```python
from build123d import *

# Parameters (mm, degrees)
ESBO_O1_W                = 9
ESBO_O1_H                = 9
ESBO_O1_R                = 8
RESSALTO_EXTRUS_O4_DEPTH = 500


with BuildPart() as part:
    # Esboço1 → Ressalto-extrusão4 (new body)
    with BuildSketch(Plane.XY):
        with BuildLine():
            Line((-4.5, 22.5), (-22.5, 22.5))
            Line((-22.5, 22.5), (-22.5, 4.5))
            Line((-22.5, 4.5), (-17.5, 4.5))
            Line((-17.5, 4.5), (-17.5, 5))
            Line((-17.5, 5), (-22, 5))
            Line((-22, 5), (-22, 12.5))
            Line((-22, 12.5), (-13.207106781, 12.5))
            Line((-13.207106781, 12.5), (-6.707685904, 6.000579123))
            ThreePointArc((-6.707685904, 6.000579123), (-9, 0), (-6.707685904, -6.000579123))
            Line((-6.707685904, -6.000579123), (-13.207106781, -12.5))
            Line((-13.207106781, -12.5), (-22, -12.5))
            Line((-22, -12.5), (-22, -5))
            Line((-22, -5), (-17.5, -5))
            Line((-17.5, -5), (-17.5, -4.5))
            Line((-17.5, -4.5), (-22.5, -4.5))
            Line((-22.5, -4.5), (-22.5, -22.5))
            Line((-22.5, -22.5), (-4.5, -22.5))
            Line((-4.5, -22.5), (-4.5, -17.5))
            Line((-4.5, -17.5), (-5, -17.5))
            Line((-5, -17.5), (-5, -22))
            Line((-5, -22), (-12.5, -22))
            Line((-12.5, -22), (-12.5, -13.207106781))
            Line((-12.5, -13.207106781), (-6.000579123, -6.707685904))
            ThreePointArc((-6.000579123, -6.707685904), (0, -9), (6.000579123, -6.707685904))
            Line((6.000579123, -6.707685904), (12.5, -13.207106781))
            Line((12.5, -13.207106781), (12.5, -22))
            Line((12.5, -22), (5, -22))
            Line((5, -22), (5, -17.5))
            Line((5, -17.5), (4.5, -17.5))
            Line((4.5, -17.5), (4.5, -22.5))
            Line((4.5, -22.5), (22.5, -22.5))
            Line((22.5, -22.5), (22.5, -4.5))
            Line((22.5, -4.5), (17.5, -4.5))
            Line((17.5, -4.5), (17.5, -5))
            Line((17.5, -5), (22, -5))
            Line((22, -5), (22, -12.5))
            Line((22, -12.5), (13.207106781, -12.5))
            Line((13.207106781, -12.5), (6.707685904, -6.000579123))
            ThreePointArc((6.707685904, -6.000579123), (9, 0), (6.707685904, 6.000579123))
            Line((6.707685904, 6.000579123), (13.207106781, 12.5))
            Line((13.207106781, 12.5), (22, 12.5))
            Line((22, 12.5), (22, 5))
            Line((22, 5), (17.5, 5))
            Line((17.5, 5), (17.5, 4.5))
            Line((17.5, 4.5), (22.5, 4.5))
            Line((22.5, 4.5), (22.5, 22.5))
            Line((22.5, 22.5), (4.5, 22.5))
            Line((4.5, 22.5), (4.5, 17.5))
            Line((4.5, 17.5), (5, 17.5))
            Line((5, 17.5), (5, 22))
            Line((5, 22), (12.5, 22))
            Line((12.5, 22), (12.5, 13.207106781))
            Line((12.5, 13.207106781), (6.000579123, 6.707685904))
            ThreePointArc((6.000579123, 6.707685904), (0, 9), (-6.000579123, 6.707685904))
            Line((-6.000579123, 6.707685904), (-12.5, 13.207106781))
            Line((-12.5, 13.207106781), (-12.5, 22))
            Line((-12.5, 22), (-5, 22))
            Line((-5, 22), (-5, 17.5))
            Line((-5, 17.5), (-4.5, 17.5))
            Line((-4.5, 17.5), (-4.5, 22.5))
        make_face()
        with Locations((17.5, 17.5)):
            Rectangle(ESBO_O1_W, ESBO_O1_H, mode=Mode.SUBTRACT)
        with Locations((-17.5, -17.5)):
            Rectangle(ESBO_O1_W, ESBO_O1_H, mode=Mode.SUBTRACT)
        with Locations((17.5, -17.5)):
            Rectangle(ESBO_O1_W, ESBO_O1_H, mode=Mode.SUBTRACT)
        with Locations((-17.5, 17.5)):
            Rectangle(ESBO_O1_W, ESBO_O1_H, mode=Mode.SUBTRACT)
        Circle(ESBO_O1_R, mode=Mode.SUBTRACT)
    extrude(amount=RESSALTO_EXTRUS_O4_DEPTH)


solid = part.part
```
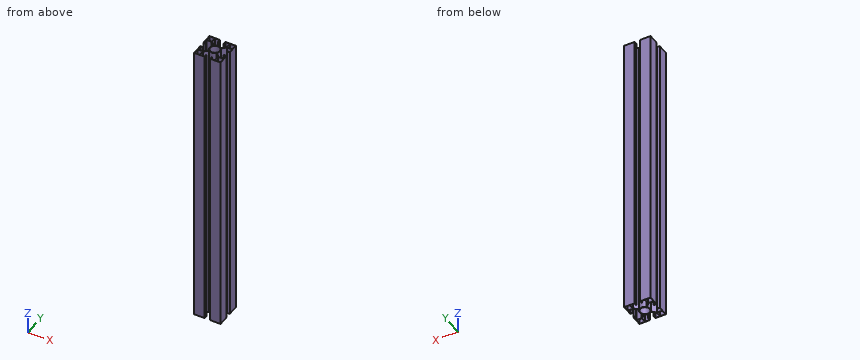
The model under review builds one solid part; all positions refer to its coordinate system, in mm. Give positions to 0.01 mm unless a question says otherwise; leave off trailing zeros. Order: outer loops, then holes, each group sorted by start corner. A loop starts at its lowest first (then second) coordinate and runs counter-clockwise, first axis right, second up. Notation, with made-up numbers: (-38, 57.5) - (-13, 57.5) arc R13 cw to (-13, 70.5) - close; hole circle Ø10 at (87.5, 78). An arc over 180 degrees is marked (long way). Use CSV: the item, a comma, the result in double quotes. Start each with the question number.
Q1. We need section A-A, the plane x = 0. Write out the cut boundary in (y, z).
Q2. To check wall thickness, follow line 1 along Y through (x, z) = (19.5, 59); line 2 along Y through (x, z) = (0, 376); line 3 along X through (y, z) = (-16, 110). State the ranges of each line that lie inside material, in increasing order. Write a range as [from, to].
Q3. Clearance check with a flat-ended pin moving along its axis: pin 1 Ø1.5 at (x, z) = (-3.5, 184) entering from -Y. State where the tip first meets the part, or that it passes through.
Q4. We need section C-C, the plane z = 127. State how many separate pieces and enclosed holes the cut face has, and give its area (3 significant figures).
Outcome:
1,outline,"(-9, 0) - (-8, 0) - (-8, 500) - (-9, 500) - close; (8, 0) - (9, 0) - (9, 500) - (8, 500) - close"
2,line 1,"y = [-22.5, -22], [-13, -12.5], [-5, -4.5], [4.5, 5], [12.5, 13], [22, 22.5]"
2,line 2,"y = [-9, -8], [8, 9]"
2,line 3,"x = [-22.5, -22], [-13, -12.5], [12.5, 13], [22, 22.5]"
3,pin 1,"stops at y = -8.57"
4,separate pieces,"1"
4,enclosed holes,"5"
4,area,"215 mm^2"
